from build123d import *

# Parameters (mm, degrees)
SKETCH4_R           = 35.56
BOSS_EXTRUDE1_DEPTH = 7.62
SKETCH5_R           = 8.89
SKETCH5_R_2         = 6.35
SKETCH7_R           = 6.35
CUT_EXTRUDE1_DEPTH  = 13.7
SKETCH8_R           = 6.35
CUT_EXTRUDE2_DEPTH  = 7.62
SKETCH10_W          = 43.18
SKETCH10_H          = 76.2
CUT_EXTRUDE3_DEPTH  = 5.08
FILLET1_R           = 5.08
FILLET2_R           = 5.08


with BuildPart() as part:
    # Sketch3 → Revolve1 (revolve)
    with BuildSketch(Plane.XY):
        Polygon((0, 0), (63.5, 0), (63.5, 76.2), (48.26, 76.2), (48.26, 127), (35.56, 127), (35.56, 63.5), (50.8, 63.5), (50.8, 12.7), (0, 12.7), align=None)
    revolve(axis=Axis((0, 12.7, 0), (0, -1, 0)))

    # Sketch4 → Boss-Extrude1 (add)
    with BuildSketch(Plane(origin=(0, 114.3, 0), x_dir=(1, 0, 0), z_dir=(0, 1, 0))):
        Circle(SKETCH4_R)
    extrude(amount=-BOSS_EXTRUDE1_DEPTH)

    # Sweep1: sweep along a path in Sketch6
    with BuildLine(Plane.XY) as sweep1_path:
        Line((15.24, 114.3), (15.24, 50.8))
        Line((15.24, 50.8), (33.02, 50.8))
        Line((33.02, 50.8), (33.02, 12.7))
    # Sketch5 → Sweep1 (sweep)
    with BuildSketch(Plane(origin=(0, 114.3, 0), x_dir=(1, 0, 0), z_dir=(0, 1, 0))):
        with Locations((15.24, 0)):
            Circle(SKETCH5_R)
        with Locations((15.24, 0)):
            Circle(SKETCH5_R_2, mode=Mode.SUBTRACT)
    sweep1 = sweep(path=sweep1_path.line, transition=Transition.RIGHT)

    # Sketch7 → Cut-Extrude1 (cut, through all)
    with BuildSketch(Plane(origin=(0, 12.7, 0), x_dir=(1, 0, 0), z_dir=(0, 1, 0))):
        with Locations((33.02, 0)):
            Circle(SKETCH7_R)
    cut_extrude1 = extrude(amount=-CUT_EXTRUDE1_DEPTH, mode=Mode.SUBTRACT)

    # Sketch8 → Cut-Extrude2 (cut)
    with BuildSketch(Plane.XZ.offset(-106.68)):
        with Locations((15.24, 0)):
            Circle(SKETCH8_R)
    cut_extrude2 = extrude(amount=-CUT_EXTRUDE2_DEPTH, mode=Mode.SUBTRACT)

    # Mirror1: Sweep1, Cut-Extrude1, Cut-Extrude2 across plane
    add(sweep1.mirror(Plane(origin=(0, 0, 0), x_dir=(0, 0, 1), z_dir=(1, 0, 0))))
    add(cut_extrude1.mirror(Plane(origin=(0, 0, 0), x_dir=(0, 0, 1), z_dir=(1, 0, 0))), mode=Mode.SUBTRACT)
    add(cut_extrude2.mirror(Plane(origin=(0, 0, 0), x_dir=(0, 0, 1), z_dir=(1, 0, 0))), mode=Mode.SUBTRACT)

    # Sketch10 → Cut-Extrude3 (cut)
    with BuildSketch(Plane.XY.offset(63.5)):
        with Locations((0, 38.1)):
            Rectangle(SKETCH10_W, SKETCH10_H)
    cut_extrude3 = extrude(amount=-CUT_EXTRUDE3_DEPTH, mode=Mode.SUBTRACT)

    # Mirror2: Cut-Extrude3 across plane
    add(cut_extrude3.mirror(Plane.XY), mode=Mode.SUBTRACT)

    # Fillet1
    fillet1_edges = [part.edges().sort_by_distance(p)[0] for p in [
        (-35.56, 114.3, 0),
    ]]
    fillet(fillet1_edges, radius=FILLET1_R)

    # Fillet2
    fillet2_edges = [part.edges().sort_by_distance(p)[0] for p in [
        (-48.26, 76.2, 0),
    ]]
    fillet(fillet2_edges, radius=FILLET2_R)


solid = part.part
Part model, mm, in its own coordinate system. A direction names the side the tool comes from. Give positions to 0.01 mm unless a question says otherwise; leave off trailing zeros. Write each loop counter-clockwise with the first axis right and the second up, starting at its lowest first coordinate (ties: lowest second). Pieces come first, ordered by that corner, then holes.
1) Two-plate mould, pull along X, no slides. Class faces 1 (the face through (1, 0, 1)), 2 (the face through (63.49, 38.63, -1.09)), 3 (the face through (46.03, 104.46, 14.5)), 4 (the face through (0, 39, 58.42)): released by +X, released by -X, zero draft, split by the parting line, or undercut.
Resolved:
face 1: zero draft
face 2: released by +X
face 3: split by the parting line
face 4: undercut
2) Cut at A-A on y = 50.8. Write the cut outline in (x, z).
Resolved:
outline: (-33.02, -8.89) - (-15.24, -8.89) arc R8.89 ccw to (-15.24, 8.89) - (-33.02, 8.89) arc R8.89 ccw to start; (-21.59, -59.72) - (-21.59, -58.42) - (21.59, -58.42) - (21.59, -59.72) arc R63.5 ccw to (21.59, 59.72) - (21.59, 58.42) - (-21.59, 58.42) - (-21.59, 59.72) arc R63.5 ccw to start; (15.24, -8.89) - (33.02, -8.89) arc R8.89 ccw to (33.02, 8.89) - (15.24, 8.89) arc R8.89 ccw to start; hole circle Ø101.6 at (0, 0); hole (-33.02, -6.35) - (-15.24, -6.35) arc R6.35 ccw to (-15.24, 6.35) - (-33.02, 6.35) arc R6.35 ccw to start; hole (15.24, -6.35) - (33.02, -6.35) arc R6.35 ccw to (33.02, 6.35) - (15.24, 6.35) arc R6.35 ccw to start
3) Probe L1, parallel to Y at x = 26, z = 0; L2, parallel to Y at x = 30, z = 0; L3, parallel to Y at x = 0, z = -18.5. List the from-to ranges inside material, lowest first.
Resolved:
L1: y = 0 to 44.45, 57.15 to 59.69, 106.68 to 114.3
L2: y = 57.15 to 59.69, 106.68 to 114.3
L3: y = 0 to 12.7, 106.68 to 114.3
4) Cut at B-B on x = 0. Write the cut outline in (y, z), then the cut area to 3 significant figures.
Resolved:
outline: (0, -58.42) - (76.2, -58.42) - (76.2, -53.34) arc R5.08 cw to (81.28, -48.26) - (127, -48.26) - (127, -35.56) - (119.38, -35.56) arc R5.08 cw to (114.3, -30.48) - (114.3, 30.48) arc R5.08 cw to (119.38, 35.56) - (127, 35.56) - (127, 48.26) - (81.28, 48.26) arc R5.08 cw to (76.2, 53.34) - (76.2, 58.42) - (0, 58.42) - close; hole (12.7, -50.8) - (63.5, -50.8) - (63.5, -35.56) - (106.68, -35.56) - (106.68, 35.56) - (63.5, 35.56) - (63.5, 50.8) - (12.7, 50.8) - close
area: 4,690 mm2
5) Pin check, flat tips, straight feed: pin 1 (5 mm diameter, centred on y = 81.5, z = 7, fed in from +X); pin 2 (3 mm diameter, centred on y = 22, z = 46.5, fed in from -X); pin 3 (10 mm diameter, centred on x = 24.5, z = 13.5, fed in from +Y). Stop position of each tip, or through.
Resolved:
pin 1: stops at x = 48.34
pin 2: stops at x = -44.8
pin 3: stops at y = 114.95
6) Which spindle directions (+Z, -Z, +X, -X, +Y, -Y) get a long thin tool onto all of the face, cutting with end or side? Do faces 5 (the face through (0, 39, -58.42)), 6 (the face through (41.232, 30.645, -3.405)), 7 (the face through (8.896, 78.886, 0.279)), 8 (the face through (-4, 127, -36)), 9 (the face through (-63.49, 38.63, 1.09)). Say none if no direction does.
Resolved:
face 5: -Z, +Y, -Y
face 6: none
face 7: +Y
face 8: +Z, -Z, +X, -X, +Y
face 9: -X, +Y, -Y
